Source: CAD feature listing. Evaluate the final solid. Frame: model axes, mm. Face numbers are marked on the shaded views. A direction names the side the tool comes from. Round coordinates to 2 decimals unless told otherwise and drop trailing zeros. Loops run counter-clockwise (first coordinate to the right, second up) from the corner with the lowest first, then second, coordinate; pieces in that order, holes last. Notation, with made-up numbers: (-12, 1) -> (3, 1) arc R18 ccw to (3, 14) -> close; hole circle Ø8 at (69, 66.5). An arc over 180 degrees is marked (long way). Return JSON: item names as keys, results as strings. Group by question number.
```python
from build123d import *

# Parameters (mm, degrees)
SKETCH006_W     = 55
SKETCH006_H     = 124
PAD002_DEPTH    = 40
POCKET004_DEPTH = 38
SKETCH008_R     = 8
POCKET005_DEPTH = 2
SKETCH009_R     = 1.1
POCKET006_DEPTH = 9
SKETCH012_R     = 2
SKETCH012_R_2   = 1
POCKET008_DEPTH = 2
SKETCH013_R     = 1.5
POCKET009_DEPTH = 2
SKETCH016_W     = 10
SKETCH016_H     = 2
POCKET011_DEPTH = 0.4
SKETCH019_W     = 51
SKETCH019_H     = 20
PAD005_DEPTH    = 14
SKETCH020_R     = 13.5
POCKET014_DEPTH = 20
SKETCH021_R     = 7
POCKET015_DEPTH = 20
SKETCH022_R     = 1.1
POCKET016_DEPTH = 10


with BuildPart() as part:
    # Sketch006 → Pad002 (new body)
    with BuildSketch(Plane.XY):
        Rectangle(SKETCH006_W, SKETCH006_H)
    extrude(amount=PAD002_DEPTH)

    # Sketch007 (on Face6 of Pad002) → Pocket004 (cut)
    with BuildSketch(Plane.XY.offset(40)):
        Polygon((-25.5, 55), (-20.5, 55), (-20.5, 60), (20.5, 60), (20.5, 55), (25.5, 55), (25.5, -55), (20.5, -55), (20.5, -60), (-20.5, -60), (-20.5, -55), (-25.5, -55), align=None)
    extrude(amount=-POCKET004_DEPTH, mode=Mode.SUBTRACT)

    # Sketch008 (on Face6 of Pocket004) → Pocket005 (cut)
    with BuildSketch(Plane.XZ.offset(62)):
        with Locations((0, 17)):
            Circle(SKETCH008_R)
    extrude(amount=-POCKET005_DEPTH, mode=Mode.SUBTRACT)

    # Sketch009 (on Face5 of Pocket005) → Pocket006 (cut)
    with BuildSketch(Plane.XY.offset(40)):
        with Locations((-24, 58.5)):
            Circle(SKETCH009_R)
        with Locations((24, 58.5)):
            Circle(SKETCH009_R)
        with Locations((24, -58.5)):
            Circle(SKETCH009_R)
        with Locations((-24, -58.5)):
            Circle(SKETCH009_R)
    extrude(amount=-POCKET006_DEPTH, mode=Mode.SUBTRACT)

    # Sketch012 (on Face2 of Pocket006) → Pocket008 (cut)
    with BuildSketch(Plane(origin=(-27.5, 0, 0), x_dir=(0, -1, 0), z_dir=(-1, 0, 0))):
        with Locations((-27.5, 25)):
            Circle(SKETCH012_R)
        with Locations((27.5, 25)):
            Circle(SKETCH012_R)
        with Locations((-36.5, 25)):
            Circle(SKETCH012_R_2)
        with Locations((36.5, 25)):
            Circle(SKETCH012_R_2)
    extrude(amount=-POCKET008_DEPTH, mode=Mode.SUBTRACT)

    # Sketch013 (on Face6 of Pocket008) → Pocket009 (cut)
    with BuildSketch(Plane.XZ.offset(62)):
        with Locations((-15, 8)):
            Circle(SKETCH013_R)
    extrude(amount=-POCKET009_DEPTH, mode=Mode.SUBTRACT)

    # Sketch016 (on Face2 of Pocket009) → Pocket011 (cut)
    with BuildSketch(Plane(origin=(-27.5, 0, 0), x_dir=(0, -1, 0), z_dir=(-1, 0, 0))):
        with Locations((-25, 9)):
            Rectangle(SKETCH016_W, SKETCH016_H)
        Polygon((20, 10), (24, 10), (24, 14), (26, 14), (26, 10), (30, 10), (30, 8), (26, 8), (26, 4), (24, 4), (24, 8), (20, 8), align=None)
    extrude(amount=-POCKET011_DEPTH, mode=Mode.SUBTRACT)

    # Sketch019 (on Face50 of Pocket011) → Pad005 (join)
    with BuildSketch(Plane.XY.offset(2)):
        with Locations((0, 5)):
            Rectangle(SKETCH019_W, SKETCH019_H)
        with Locations((0, -45)):
            Rectangle(SKETCH019_W, SKETCH019_H)
    extrude(amount=PAD005_DEPTH)

    # Sketch020 (on Face53 of Pad005) → Pocket014 (cut)
    with BuildSketch(Plane.XZ.offset(5)):
        with Locations((0, 17)):
            Circle(SKETCH020_R)
    extrude(amount=-POCKET014_DEPTH, mode=Mode.SUBTRACT)

    # Sketch021 (on Face55 of Pad005) → Pocket015 (cut)
    with BuildSketch(Plane(origin=(0, -35, 0), x_dir=(-1, 0, 0), z_dir=(0, 1, 0))):
        with Locations((0, 17)):
            Circle(SKETCH021_R)
    extrude(amount=-POCKET015_DEPTH, mode=Mode.SUBTRACT)

    # Sketch022 (on Face60 of Pocket015) → Pocket016 (cut)
    with BuildSketch(Plane.XY.offset(16)):
        with Locations((-20, 5)):
            Circle(SKETCH022_R)
        with Locations((20, 5)):
            Circle(SKETCH022_R)
        with Locations((-20, -45)):
            Circle(SKETCH022_R)
        with Locations((20, -45)):
            Circle(SKETCH022_R)
    extrude(amount=-POCKET016_DEPTH, mode=Mode.SUBTRACT)


with BuildPart() as part_1:
    # Body002 placement: moved
    add(part.part.moved(Location((0, 0, -2))))


solid = part_1.part
```
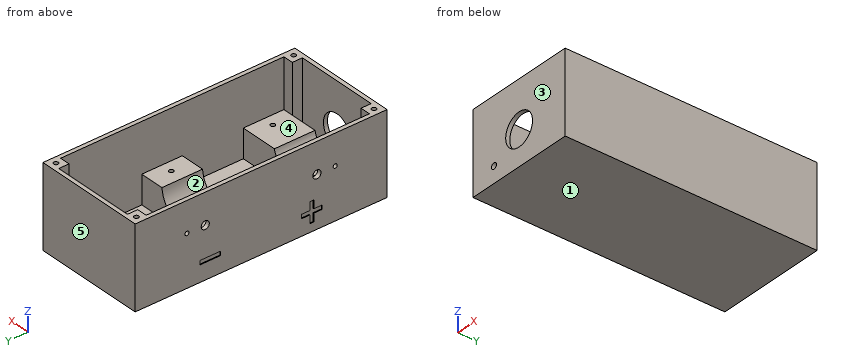
(1) Cut plane C-C (y = -33). Return loops of the section in (x, z).
(2) Ray query, line 1 (Y direction, x = -17.5, z = 9); line 2 (Y direction, x = 24, z = 31); line 3 (Z direction, x = 0, y = -61). Return the intervals inside material, ascending.
(3) Mould query, pull axis Y, two halves, no side actions, for the marked faces 1, 2 and 3. Classes: released by +Y, released by -Y, zero draft, split by the parting line, or undercut.
(4) Cut plane D-D (x = -1.5). Return loops of the section in (y, z), and give its area (3 significant figures).
(5) Pin query (flat end, axial travel): pin 1 (2 mm diameter, centred on x = 20, y = -45, fed in from +Z); pin 2 (6 mm diameter, centred on x = -9, y = -28.5, fed in from +Z); pin 3 (4 mm diameter, centred on x = 1, z = 19.5, fed in from -Y). Return the tip coordinate at first contact, or that it passes through.
(6) Cut plane A-A (x = -15). Return loops of the section in (y, z), and give its area (3 significant figures).
(7) Set-up query: the marked faces 4 and 5. Return all of +Z, -Z, +X, -X, +Y, -Y with unobstructed straight access to the full face (end or side cutting, diameter ignored); none if empty.
(8) Cut plane B-B (z = 32). Return loops of the section in (x, y).
Answers follow:
{
 "1": {"outline": "(-27.5, -2) -> (27.5, -2) -> (27.5, 38) -> (25.5, 38) -> (25.5, 0) -> (-25.5, 0) -> (-25.5, 38) -> (-27.5, 38) -> close"},
 "2": {"line 1": "-62 to -60, -55 to -35, -5 to 15, 60 to 62", "line 2": "-62 to -59.6, -57.4 to -55, 55 to 57.4, 59.6 to 62", "line 3": "-2 to 7, 23 to 38"},
 "3": {"face 1": "zero draft", "face 2": "undercut", "face 3": "released by -Y"},
 "4": {"outline": "(-62, -2) -> (62, -2) -> (62, 38) -> (60, 38) -> (60, 0) -> (15, 0) -> (15, 1.58) -> (-5, 1.58) -> (-5, 0) -> (-35, 0) -> (-35, 8.16) -> (-55, 8.16) -> (-55, 0) -> (-60, 0) -> (-60, 7.14) -> (-62, 7.14) -> close; (-62, 22.86) -> (-60, 22.86) -> (-60, 38) -> (-62, 38) -> close", "area": "563 mm^2"},
 "5": {"pin 1": "z = 4", "pin 2": "z = 0", "pin 3": "y = 60"},
 "6": {"outline": "(-62, -2) -> (62, -2) -> (62, 38) -> (60, 38) -> (60, 0) -> (15, 0) -> (15, 14) -> (-5, 14) -> (-5, 0) -> (-35, 0) -> (-35, 14) -> (-55, 14) -> (-55, 0) -> (-60, 0) -> (-60, 4.5) -> (-62, 4.5) -> close; (-62, 7.5) -> (-60, 7.5) -> (-60, 38) -> (-62, 38) -> close", "area": "954 mm^2"},
 "7": {"face 4": "+Z", "face 5": "+Z, -Z, +X, -X, +Y"},
 "8": {"outline": "(-27.5, -62) -> (27.5, -62) -> (27.5, 62) -> (-27.5, 62) -> close; hole (-25.5, -55) -> (-20.5, -55) -> (-20.5, -60) -> (20.5, -60) -> (20.5, -55) -> (25.5, -55) -> (25.5, 55) -> (20.5, 55) -> (20.5, 60) -> (-20.5, 60) -> (-20.5, 55) -> (-25.5, 55) -> close; hole circle Ø2.2 at (-24, -58.5); hole circle Ø2.2 at (-24, 58.5); hole circle Ø2.2 at (24, -58.5); hole circle Ø2.2 at (24, 58.5)"}
}
